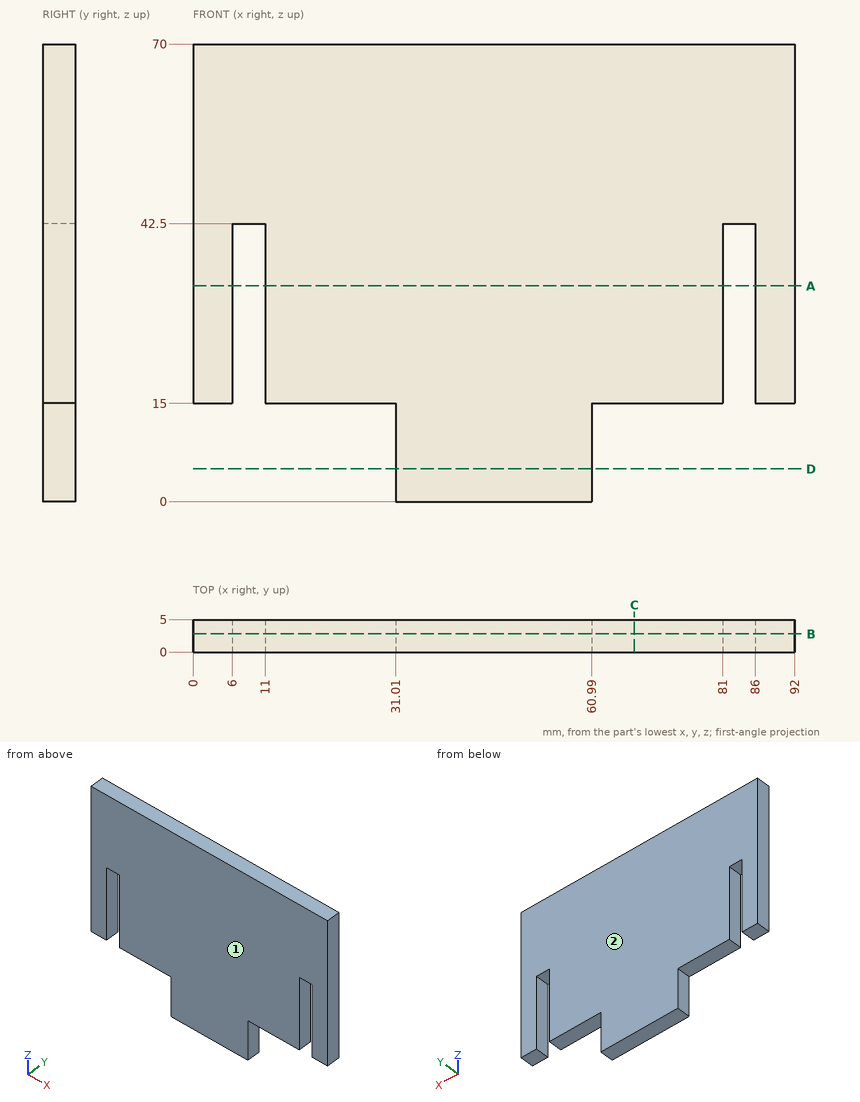
Answer from the drawing. Dimensions are ordinates in mm from the lowest x, y and z of the part. Coordinates: 2 decimals unless noted, no trailing zeros. Order: outer loops, then holes, each group sorted by start corner. A loop starts at its lowest first (then second) coordinate and runs counter-clockwise, first axis right, second up. Notation, with made-up numbers: (74, -30) - (85, -30) arc R20 cw to (85, 7) - close; hole circle Ø7 at (-27.5, 19.5). An arc over 180 degrees is marked (long way). Answer as a JSON object with one key per item and string values. Group by question number.
Item 1: Section A-A (z = 33) is taken. Give the vertices of the cut face in (x, y), plus the area to 3 significant figures.
Item 2: Section B-B (y = 2.8) is taken. Give the vertices of the cut face in (x, z).
Item 3: The mould has two halves that part along Y. Classify the marked faces 1 and 2: +Y half, -Y half, draft (parallel to the pull), parting line (faces both ways), or undercut.
Item 4: Section D-D (z = 5) is taken. Give the vertices of the cut face in (x, y).
Item 5: Consider probe 1 along X at (y, z) = (1.5, 23); probe 2 along Z at (x, y) = (16, 0.3); probe 3 along X at (y, z) = (4.2, 7.5). Determine where each line is inside the solid, lowest interval first. Write a range as from..to.
Item 6: Section C-C (x = 67.5) is taken. Give the vertices of the cut face in (y, z).
Item 7: Flat-ended cylindrical pins translate along their axes: P1, Ø1.5, axis at x = 4.5, y = 1.5, coming from the -Z side; P2, Ø1.5, axis at x = 7.5, y = 2.5, coming from the -Z side; P3, Ø2.5, axis at y = 1.5, z = 5, coming from the +X side. Find the tip coordinate at first contact, or state that the pin passes through.
Results are:
{
 "1": {"outline": "(0, 0) - (6, 0) - (6, 5) - (0, 5) - close; (11, 0) - (81, 0) - (81, 5) - (11, 5) - close; (86, 0) - (92, 0) - (92, 5) - (86, 5) - close", "area": "410 mm^2"},
 "2": {"outline": "(0, 15) - (6, 15) - (6, 42.5) - (11, 42.5) - (11, 15) - (31.01, 15) - (31.01, 0) - (60.99, 0) - (60.99, 15) - (81, 15) - (81, 42.5) - (86, 42.5) - (86, 15) - (92, 15) - (92, 70) - (0, 70) - close"},
 "3": {"face 1": "-Y half", "face 2": "+Y half"},
 "4": {"outline": "(31.01, 0) - (60.99, 0) - (60.99, 5) - (31.01, 5) - close"},
 "5": {"probe 1": "x = 0..6, 11..81, 86..92", "probe 2": "z = 15..70", "probe 3": "x = 31.01..60.99"},
 "6": {"outline": "(0, 15) - (5, 15) - (5, 70) - (0, 70) - close"},
 "7": {"P1": "stops at z = 15", "P2": "stops at z = 42.5", "P3": "stops at x = 60.99"}
}
